Verification items for the finished model (mm, model axes). A direction names the side the tool comes from. Round coordinates to 2 decimals unless told otherwise and drop trailing zeros. Order: outer loops, then holes, each group sorted by start corner. A loop starts at its lowest first (then second) coordinate and runs counter-clockwise, first axis right, second up. Notation, with made-up numbers: M 82,54 L 136,54 A7 cw 136,64 Z; hole C 32.5,-35.5 d9. An arc over 180 degrees is marked long. Use CSV: the item, a comma, the result in double quotes. Start each with the question number.
Q1. Sectioned sample at C-C (y = 3.75). Enter the section's corners in (x, z) (3 decimals).
Q2. Set-up check for faces 1 (the face through (10, 2, 50)), 2 (the face through (83, 2, 20)), 3 (the face through (20, 2, 3)): record each of +Z, -Z, +X, -X, +Y, -Y from which the full face is reachable in a straight line by a thin tool's end or side.
Q3. Sectioned sample at D-D (z = 41). Enter the section's corners in (x, y), and give its area (3 significant figures).
Q4. Scan lines: line 1 (Z direction, x = 10, y = 3.65) (3 decimals); line 2 (X direction, y = 3.2, z = 3); line 3 (Z direction, x = 85, y = 3.5). Record each from-to range of solid material in increasing order.
Q5. Sectioned sample at B-B (x = 12). Enter the section's corners in (y, z).
Q6. Mould release check, pull along X, two halves, no side actions. Record for faces 4 (the face through (31, 2, 40)), 5 (the face through (75, 2, 4)), 6 (the face through (94.43, 2.46, 19.4)): +X half, -X half, draft (parallel to the pull), parting line (faces both ways), or undercut.
Q7. Sectioned sample at A-A (x = 85). Enter the section's corners in (y, z), and give its area (3 significant figures).
Q8. Gauge pin test, flat ends, axial feed: pin 1 Ø3 at (y, z) = (4, 28) entering from +X; pin 2 Ø1.5 at (x, y) = (81, 4) entering from +Z; pin 3 Ø2.5 at (y, z) = (2.5, 44) entering from +X. Record the tip position at first contact, or that the pin passes through.
Autodesk Inventor part; units mm, degrees
ref_plane "YZ Plane" through (0, 0, 0) normal (1, 0, 0) x (0, 1, 0)
ref_plane "XZ Plane" through (0, 0, 0) normal (0, 1, 0) x (-1, 0, 0)
ref_plane "XY Plane" through (0, 0, 0) normal (0, 0, 1) x (1, 0, 0)
sketch "Sketch1" plane through (0, 0, 0) normal (0, 1, 0) x (-1, 0, 0)
  line L0 (0, 2) -> (0, 48)
  line L1 (-2, 50) -> (-18, 50)
  line L2 (-20, 48) -> (-20, 42)
  line L3 (-22, 40) -> (-40, 40)
  line L4 (-2, 0) -> (-20, 0)
  line L5 (-20, 0) -> (-20, 6)
  line L6 (-24, 10) -> (-71, 10)
  line L7 (-75, 6) -> (-75, 2)
  line L8 (-77, 0) -> (-93, 0)
  line L9 (-95, 2) -> (-95, 18)
  arc A0 (-72.8634, 20) -> (-41.7764, 38.9189) centre (-72.8634, 55) ccw
  arc A1 (-40, 40) -> (-41.7764, 38.9189) centre (-40, 38) ccw
  line L10 (-93, 20) -> (-72.8634, 20)
  arc A2 (0, 48) -> (-2, 50) centre (-2, 48) ccw
  arc A3 (-2, 0) -> (0, 2) centre (-2, 2) ccw
  arc A4 (-18, 50) -> (-20, 48) centre (-18, 48) ccw
  arc A5 (-22, 40) -> (-20, 42) centre (-22, 42) ccw
  arc A6 (-77, 0) -> (-75, 2) centre (-77, 2) ccw
  arc A7 (-95, 2) -> (-93, 0) centre (-93, 2) ccw
  arc A8 (-93, 20) -> (-95, 18) centre (-93, 18) ccw
  arc A9 (-20, 6) -> (-24, 10) centre (-24, 6) ccw
  arc A10 (-71, 10) -> (-75, 6) centre (-71, 6) ccw
  circle A11 centre (-10, 40) radius 3.225
  circle A12 centre (-10, 10) radius 5.25
  circle A13 centre (-35, 20) radius 2.5
  circle A14 centre (-85, 10) radius 5.25
  point P0 (0, 0)
  point P1 (0, 50)
  point P2 (-20, 50)
  point P3 (-20, 40)
  point P4 (-20, 10)
  point P5 (-75, 10)
  point P6 (-75, 0)
  point P7 (-95, 0)
  point P8 (-95, 20)
  dimension "d0" = 50
  dimension "d1" = 20
  dimension "d2" = 10
  dimension "d3" = 20
  dimension "d4" = 20
  dimension "d5" = 10
  dimension "d6" = 55
  dimension "d7" = 20
  dimension "d8" = 20
  dimension "d9" = 70
  dimension "d11" = 4
  dimension "d12" = 2
  dimension "d13" = 2
  dimension "d14" = 4
  dimension "d15" = 6.45
  dimension "d16" = 10.5
  dimension "d17" = 30
  dimension "d18" = 10
  dimension "d19" = 10
  dimension "d20" = 10
  dimension "d21" = 5
  dimension "d22" = 25
  dimension "d25" = 10.5
  dimension "d26" = 10
extrude "Extrusion1" add sketch "Sketch1" along normal blind 5
properties part number "Barrel Support" material "Wood (Walnut)"
Verdict:
1,outline,"M 0,2 A2 ccw 2,0 L 20,0 L 20,6 A4 cw 24,10 L 71,10 A4 cw 75,6 L 75,2 A2 ccw 77,0 L 93,0 A2 ccw 95,2 L 95,18 A2 ccw 93,20 L 72.863,20 A35 cw 41.776,38.919 A2 ccw 40,40 L 22,40 A2 cw 20,42 L 20,48 A2 ccw 18,50 L 2,50 A2 ccw 0,48 Z; hole C 10,10 d10.5; hole C 10,40 d6.45; hole C 35,20 d5; hole C 85,10 d10.5"
2,face 1,"+Z, +X, -X, +Y, -Y"
2,face 2,"+Z, +X, +Y, -Y"
2,face 3,"-Z, +Y, -Y"
3,outline,"M 0,0 L 6.93,0 L 6.93,5 L 0,5 Z; M 13.07,0 L 20.27,0 L 20.27,5 L 13.07,5 Z"
3,area,"70.7 mm²"
4,line 1,"z = 0 to 4.75, 15.25 to 36.775, 43.225 to 50"
4,line 2,"x = 0 to 20, 75 to 95"
4,line 3,"z = 0 to 4.75, 15.25 to 20"
5,outline,"M 0,0 L 5,0 L 5,5.15 L 0,5.15 Z; M 0,14.85 L 5,14.85 L 5,37.47 L 0,37.47 Z; M 0,42.53 L 5,42.53 L 5,50 L 0,50 Z"
6,face 4,"draft"
6,face 5,"undercut"
6,face 6,"+X half"
7,outline,"M 0,0 L 5,0 L 5,4.75 L 0,4.75 Z; M 0,15.25 L 5,15.25 L 5,20 L 0,20 Z"
7,area,"47.5 mm²"
8,pin 1,"stops at x = 52.55"
8,pin 2,"stops at z = 20"
8,pin 3,"stops at x = 20"
